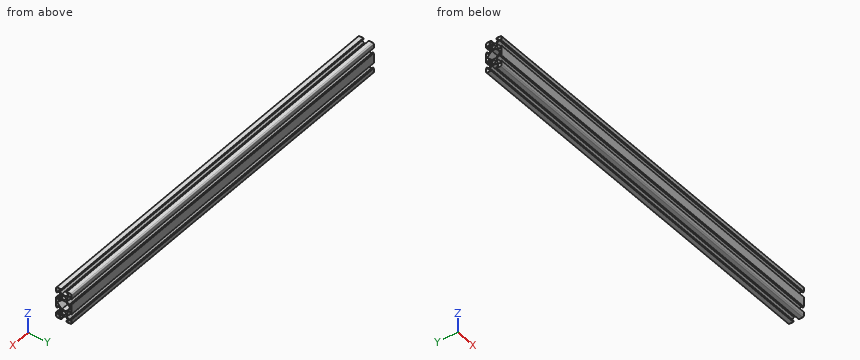
```python
from build123d import *

# Parameters (mm, degrees)
SKETCH11_R               = 2.5
F_20_X_40_X_T1_5_1_DEPTH = 508


with BuildPart() as part:
    # Sketch11 → 铝型材 20 X 40 X T1.5(1) (new body)
    with BuildSketch(Plane.YZ):
        with BuildLine():
            Line((-3.6, 10), (-3.6, 9.5))
            Line((-3.6, 9.5), (-3.1, 9.5))
            Line((-3.1, 9.5), (-3.1, 8.5))
            Line((-3.1, 8.5), (-5.5, 8.5))
            Line((-5.5, 8.5), (-5.5, 6.65))
            Line((-5.5, 6.65), (-2.75, 3.9))
            Line((-2.75, 3.9), (2.75, 3.9))
            Line((2.75, 3.9), (5.5, 6.65))
            Line((5.5, 6.65), (5.5, 8.5))
            Line((5.5, 8.5), (3.1, 8.5))
            Line((3.1, 8.5), (3.1, 9.5))
            Line((3.1, 9.5), (3.6, 9.5))
            Line((3.6, 9.5), (3.6, 10))
            Line((3.6, 10), (8.5, 10))
            ThreePointArc((8.5, 10), (9.560660172, 9.560660172), (10, 8.5))
            Line((10, 8.5), (10, 3.6))
            Line((10, 3.6), (9.5, 3.6))
            Line((9.5, 3.6), (9.5, 3.1))
            Line((9.5, 3.1), (8.5, 3.1))
            Line((8.5, 3.1), (8.5, 5.5))
            Line((8.5, 5.5), (6.65, 5.5))
            Line((6.65, 5.5), (3.9, 2.75))
            Line((3.9, 2.75), (3.9, -2.75))
            Line((3.9, -2.75), (6.65, -5.5))
            Line((6.65, -5.5), (8.5, -5.5))
            Line((8.5, -5.5), (8.5, -3.1))
            Line((8.5, -3.1), (9.5, -3.1))
            Line((9.5, -3.1), (9.5, -3.6))
            Line((9.5, -3.6), (10, -3.6))
            Line((10, -3.6), (10, -16.4))
            Line((10, -16.4), (9.5, -16.4))
            Line((9.5, -16.4), (9.5, -16.9))
            Line((9.5, -16.9), (8.5, -16.9))
            Line((8.5, -16.9), (8.5, -14.5))
            Line((8.5, -14.5), (6.65, -14.5))
            Line((6.65, -14.5), (3.9, -17.25))
            Line((3.9, -17.25), (3.9, -22.75))
            Line((3.9, -22.75), (6.65, -25.5))
            Line((6.65, -25.5), (8.5, -25.5))
            Line((8.5, -25.5), (8.5, -23.1))
            Line((8.5, -23.1), (9.5, -23.1))
            Line((9.5, -23.1), (9.5, -23.6))
            Line((9.5, -23.6), (10, -23.6))
            Line((10, -23.6), (10, -28.5))
            ThreePointArc((10, -28.5), (9.560660172, -29.560660172), (8.5, -30))
            Line((8.5, -30), (3.6, -30))
            Line((3.6, -30), (3.6, -29.5))
            Line((3.6, -29.5), (3.1, -29.5))
            Line((3.1, -29.5), (3.1, -28.5))
            Line((3.1, -28.5), (5.5, -28.5))
            Line((5.5, -28.5), (5.5, -26.65))
            Line((5.5, -26.65), (2.75, -23.9))
            Line((2.75, -23.9), (-2.75, -23.9))
            Line((-2.75, -23.9), (-5.5, -26.65))
            Line((-5.5, -26.65), (-5.5, -28.5))
            Line((-5.5, -28.5), (-3.1, -28.5))
            Line((-3.1, -28.5), (-3.1, -29.5))
            Line((-3.1, -29.5), (-3.6, -29.5))
            Line((-3.6, -29.5), (-3.6, -30))
            Line((-3.6, -30), (-8.5, -30))
            ThreePointArc((-8.5, -30), (-9.560660172, -29.560660172), (-10, -28.5))
            Line((-10, -28.5), (-10, -23.6))
            Line((-10, -23.6), (-9.5, -23.6))
            Line((-9.5, -23.6), (-9.5, -23.1))
            Line((-9.5, -23.1), (-8.5, -23.1))
            Line((-8.5, -23.1), (-8.5, -25.5))
            Line((-8.5, -25.5), (-6.65, -25.5))
            Line((-6.65, -25.5), (-3.9, -22.75))
            Line((-3.9, -22.75), (-3.9, -17.25))
            Line((-3.9, -17.25), (-6.65, -14.5))
            Line((-6.65, -14.5), (-8.5, -14.5))
            Line((-8.5, -14.5), (-8.5, -16.9))
            Line((-8.5, -16.9), (-9.5, -16.9))
            Line((-9.5, -16.9), (-9.5, -16.4))
            Line((-9.5, -16.4), (-10, -16.4))
            Line((-10, -16.4), (-10, -3.6))
            Line((-10, -3.6), (-9.5, -3.6))
            Line((-9.5, -3.6), (-9.5, -3.1))
            Line((-9.5, -3.1), (-8.5, -3.1))
            Line((-8.5, -3.1), (-8.5, -5.5))
            Line((-8.5, -5.5), (-6.65, -5.5))
            Line((-6.65, -5.5), (-3.9, -2.75))
            Line((-3.9, -2.75), (-3.9, 2.75))
            Line((-3.9, 2.75), (-6.65, 5.5))
            Line((-6.65, 5.5), (-8.5, 5.5))
            Line((-8.5, 5.5), (-8.5, 3.1))
            Line((-8.5, 3.1), (-9.5, 3.1))
            Line((-9.5, 3.1), (-9.5, 3.6))
            Line((-9.5, 3.6), (-10, 3.6))
            Line((-10, 3.6), (-10, 8.5))
            ThreePointArc((-10, 8.5), (-9.560660172, 9.560660172), (-8.5, 10))
            Line((-8.5, 10), (-3.6, 10))
        make_face()
        Circle(SKETCH11_R, mode=Mode.SUBTRACT)
        with Locations((0, -20)):
            Circle(SKETCH11_R, mode=Mode.SUBTRACT)
        Polygon((8.85, -10), (2.75, -3.9), (-2.75, -3.9), (-8.85, -10), (-2.75, -16.1), (2.75, -16.1), align=None, mode=Mode.SUBTRACT)
    extrude(amount=F_20_X_40_X_T1_5_1_DEPTH)


solid = part.part
```
Input: part model. Units: mm. Frame: model coordinates. Round coordinates to 2 decimals unless told otherwise and drop trailing zeros. One line per question, with ' | ' between items. Start each with the question number.
1) Cut plane A-A, the plane x = 348. Give the number of separate pieces and of enclosed holes in the cut face, then the cut area to 3 significant figures.
2) Contact query for flat-ended pins moving along their axis: P1, Ø3, axis at x = 215.5, z = -18.5, coming from the -Y side; P2, Ø5, axis at x = 203, z = -19, coming from the -Y side; P3, Ø1.6, axis at x = 317, z = -1, coming from the -Y side. Output: stop coordinate, or through.
3) Ray query, probe 1 along Z at (x, y) = (364.5, 0); probe 2 along Z at (x, y) = (389.5, -9); probe 3 along Z at (x, y) = (139, -8.75). Return the intervals inside material, ascending.
Worked out:
1) separate pieces: 1 | enclosed holes: 3 | area: 300 mm^2
2) P1: stops at y = -4.15 | P2: stops at y = -9.5 | P3: stops at y = -3.9
3) probe 1: z = -23.9 to -22.5, -17.5 to -16.1, -3.9 to -2.5, 2.5 to 3.9 | probe 2: z = -29.91 to -23.1, -16.9 to -3.1, 3.1 to 9.91 | probe 3: z = -29.98 to -23.1, -16.9 to -10.1, -9.9 to -3.1, 3.1 to 9.98
